Autodesk Inventor part; units mm, degrees
ref_plane "YZ Plane" through (0, 0, 0) normal (1, 0, 0) x (0, 1, 0)
ref_plane "XZ Plane" through (0, 0, 0) normal (0, 1, 0) x (-1, 0, 0)
ref_plane "XY Plane" through (0, 0, 0) normal (0, 0, 1) x (1, 0, 0)
sketch "Sketch1" plane through (0, 0, 0) normal (0, 1, 0) x (-1, 0, 0)
  line L0 (-30, 75) -> (30, 75)
  line L1 (30, 75) -> (30, -75)
  line L2 (30, -75) -> (-30, -75)
  line L3 (-30, -75) -> (-30, 75)
  line L4 (30, 75) -> (25, 75)
  line L5 (25, 75) -> (25, 70)
  line L6 (25, 70) -> (30, 70)
  line L7 (30, 70) -> (30, 75)
  line L8 (-30, 75) -> (-25, 75)
  line L9 (-25, 75) -> (-25, 70)
  line L10 (-25, 70) -> (-30, 70)
  line L11 (-30, 70) -> (-30, 75)
  line L12 (30, -75) -> (25, -75)
  line L13 (25, -75) -> (25, -70)
  line L14 (25, -70) -> (30, -70)
  line L15 (30, -70) -> (30, -75)
  line L16 (-30, -75) -> (-25, -75)
  line L17 (-25, -75) -> (-25, -70)
  line L18 (-25, -70) -> (-30, -70)
  line L19 (-30, -70) -> (-30, -75)
  circle A0 centre (25, 70) radius 1.4
  circle A1 centre (-25, 70) radius 1.4
  circle A2 centre (25, -70) radius 1.4
  circle A3 centre (-25, -70) radius 1.4
  line L20 (-9.515, 11.025) -> (9.515, 11.025)
  line L21 (9.515, 11.025) -> (9.515, -11.025)
  line L22 (9.515, -11.025) -> (-9.515, -11.025)
  line L23 (-9.515, -11.025) -> (-9.515, 11.025)
  line L24 (-9.515, 11.025) -> (9.515, -11.025) construction
  line L25 (9.515, 11.025) -> (-9.515, -11.025) construction
  line L26 (-9.515, -11.025) -> (-7.015, -11.025)
  line L27 (-7.015, -11.025) -> (-7.015, -8.525)
  line L28 (-7.015, -8.525) -> (-9.515, -8.525)
  line L29 (-9.515, -8.525) -> (-9.515, -11.025)
  line L30 (-9.515, 11.025) -> (-7.015, 11.025)
  line L31 (-7.015, 11.025) -> (-7.015, 8.525)
  line L32 (-7.015, 8.525) -> (-9.515, 8.525)
  line L33 (-9.515, 8.525) -> (-9.515, 11.025)
  circle A4 centre (-7.015, 8.525) radius 1.5
  circle A5 centre (-7.015, -8.525) radius 1.5
  line L34 (9.515, 0) -> (8.515, 0)
  line L35 (6.515, -11.025) -> (10.515, -11.025)
  line L36 (10.515, -11.025) -> (10.515, 11.025)
  line L37 (10.515, 11.025) -> (6.515, 11.025)
  line L38 (6.515, 11.025) -> (6.515, -11.025)
  line L39 (6.515, -11.025) -> (10.515, 11.025) construction
  line L40 (10.515, -11.025) -> (6.515, 11.025) construction
  line L41 (0, -75) -> (-20, -75)
  line L42 (0, -75) -> (20, -75)
  point P0 (0, 0)
  point P1 (0, 0)
  dimension "d0" = 60
  dimension "d1" = 150
  dimension "d2" = 5
  dimension "d3" = 5
  dimension "d4" = 5
  dimension "d5" = 5
  dimension "d6" = 5
  dimension "d8" = 5
  dimension "d10" = 2.8
  dimension "d11" = 2.8
  dimension "d12" = 19.03
  dimension "d13" = 22.05
  dimension "d14" = 2.5
  dimension "d15" = 2.5
  dimension "d16" = 2.5
  dimension "d17" = 2.5
  dimension "d18" = 3
  dimension "d19" = 3
  dimension "d20" = 1
  dimension "d21" = 4
extrude "Extrusion1" add sketch "Sketch1" along normal blind 3 contours L0 L9 A1 L10 L3 | L0 L5 A0 L6 L1 L14 A2 L13 L2 L17 A3 L18 L3 L10 A1 L9 | L0 L1 L6 A0 L5 | L18 A3 L17 L2 L3 | L1 L2 L13 A2 L14 | L20 L31 A4 L32 L23 | L20 L38 L22 L27 A5 L28 L23 L32 A4 L31 | L20 L21 L22 L38 | L28 A5 L27 L22 L23 | L37 L36 L35 L21
fillet "Fillet1" radius 2.8 1 edges at (30, 1.5, 75)
fillet "Fillet2" radius 2.8 1 edges at (-30, 1.5, 75)
fillet "Fillet3" radius 2.8 1 edges at (-30, 1.5, -75)
fillet "Fillet4" radius 2.8 1 edges at (30, 1.5, -75)
properties part number "MatTren"
The listing builds one solid part. Answer for the finished solid, in the listing's coordinates (mm). Coordinates: 2 decimals unless noted, no trailing zeros. Order: outer loops, then holes, each group sorted by start corner. A loop starts at its lowest first (then second) coordinate and runs counter-clockwise, first axis right, second up.
Q1. A cutting plane is placed at B-B, the plane z = 70. Write down the section's boundary in (x, y).
Q2. For a pull along Z with two mould halves and no side action, classify faces 1 (the face through (7.21, 1.479, -10.012)), 2 (the face through (-30, 1, 1)), 3 (the face through (-29.16, 1.52, -74.2)), 4 (the face through (-25.65, 1.48, -68.76)) as pulls with the +Z half, pulls with the -Z half, needs draft (parallel to the pull), parting line crosses it, or undercut.
Q3. A cutting plane is placed at A-A, the plane x = -25. Write down the section's boundary in (y, z), and give its area (3 significant figures).
Q4. Given P1, Ø5, axis at x = 7.015, z = -8.525, coming from the -Y side; P2, Ø2.5, axis at x = 7.015, z = 8.525, coming from the +Y side, each flat-ended and moving along its own axis, determine where each tip first touches the part or whether it passes through.
Q5. Consider line 1 (Z direction, x = -25, y = 1.65); line 2 (X direction, y = 0.75, z = 70); line 3 (Z direction, x = -26, y = 1.1). Determine where each line is inside the solid, lowest interval first.
Answers follow:
1. outline: (-30, 0) - (-26.4, 0) - (-26.4, 3) - (-30, 3) - close; (-23.6, 0) - (23.6, 0) - (23.6, 3) - (-23.6, 3) - close; (26.4, 0) - (30, 0) - (30, 3) - (26.4, 3) - close
2. face 1: undercut
2. face 2: needs draft
2. face 3: pulls with the -Z half
2. face 4: undercut
3. outline: (0, -75) - (3, -75) - (3, -71.4) - (0, -71.4) - close; (0, -68.6) - (3, -68.6) - (3, 68.6) - (0, 68.6) - close; (0, 71.4) - (3, 71.4) - (3, 75) - (0, 75) - close
3. area: 433 mm2
4. P1: stops at y = 0
4. P2: passes through
5. line 1: z = -75 to -71.4, -68.6 to 68.6, 71.4 to 75
5. line 2: x = -30 to -26.4, -23.6 to 23.6, 26.4 to 30
5. line 3: z = -75 to -70.98, -69.02 to 69.02, 70.98 to 75
